Read the model definition and answer for the solid it produces. Units are mm, in the model's axes. Face numbers are marked on the shaded views. A direction names the side the tool comes from. Give positions to 0.01 mm unless a question says otherwise; leave off trailing zeros. Loops run counter-clockwise (first coordinate to the right, second up) from the corner with the lowest first, then second, coordinate; pieces in that order, holes last. Notation, with made-up numbers: (59.5, 16) -> (106.5, 16) arc R23 ccw to (106.5, 32) -> close; hole circle Ø9 at (-7.5, 67). An arc over 180 degrees is marked (long way). Write each question's results on one line, items separated by ' | '. Start each with the question number.
Item 1: Each of these flat-tipped pins is pushed along its axis until it touches: P1, Ø2, axis at x = 1.5, z = 2.5, coming from the +Y side; P2, Ø0.5, axis at y = 2.5, z = -3.5, coming from the -X side. Where does it stop, or does it pass through?
Item 2: Find the intervals of material crossed by line 1 (Z direction, x = 4, y = 1.85); line 2 (Z direction, x = -1, y = 2.45); line 3 (Y direction, x = 1.75, z = -2.5), in increasing order.
Item 3: Section A-A on z = -2 is taken. Write down the section's boundary in (x, y).
Item 4: Section B-B on y = 2.3 is taken. Write down the section's boundary in (x, z), and give its area (3 significant figures).
Item 5: Which of the six approach directions +Z, -Z, +X, -X, +Y, -Y give full straight-line access (tool end or side, diameter ignored) to the marked faces 1 and 2?
Item 6: Section C-C on x = 4 is taken. Write down the section's boundary in (y, z).
Item 7: Section D-D on z = 2.5 is taken. Write down the section's boundary in (x, y), and give its area (3 significant figures).
Item 8: Determine the mould class of the marked faces 3, 4 and 5 for opening direction Z: +Z half, -Z half, draft (parallel to the pull), parting line (faces both ways), or undercut.
Autodesk Inventor part; units mm, degrees
ref_plane "YZ Plane" through (0, 0, 0) normal (1, 0, 0) x (0, 1, 0)
ref_plane "XZ Plane" through (0, 0, 0) normal (0, 1, 0) x (-1, 0, 0)
ref_plane "XY Plane" through (0, 0, 0) normal (0, 0, 1) x (1, 0, 0)
sketch "草圖1" plane through (0, 0, 0) normal (0, 1, 0) x (-1, 0, 0)
  line L0 (2.7779, 3.5245) -> (-4.7221, 3.5245)
  line L1 (-4.7221, 3.5245) -> (-4.7221, -6.4755)
  line L2 (-4.7221, -6.4755) -> (2.7779, -6.4755)
  line L3 (2.7779, -6.4755) -> (2.7779, 3.5245)
  line L4 (1.1026, 3.5245) -> (1.1026, -6.4755)
  line L5 (1.1026, 0.7245) -> (-4.7221, 0.7245)
  line L6 (1.1026, -0.0755) -> (-4.7221, -0.0755)
  line L7 (1.1026, -2.8755) -> (-4.7221, -2.8755)
  line L8 (1.1026, -3.6755) -> (-4.7221, -3.6755)
  line L9 (1.1026, -1.4755) -> (-4.7221, -1.4755)
  line L10 (0.6975, -1.6358) -> (-3.8571, -1.6358)
  line L11 (-3.8571, -1.6358) -> (-3.8571, -2.7441)
  line L12 (-3.8571, -2.7441) -> (0.6975, -2.7441)
  line L13 (0.6975, -2.7441) -> (0.6975, -1.6358)
  line L14 (0.6975, -1.3152) -> (-3.8571, -1.3152)
  line L15 (-3.8571, -1.3152) -> (-3.8571, -0.207)
  line L16 (-3.8571, -0.207) -> (0.6975, -0.207)
  line L17 (0.6975, -0.207) -> (0.6975, -1.3152)
  line L18 (1.4446, 3.5245) -> (1.4446, -6.4755)
  line L19 (1.2626, 3.5245) -> (1.2626, -6.4755)
  line L20 (1.6046, 3.5245) -> (1.6046, -6.4755)
  line L21 (1.9385, 3.5245) -> (1.9385, -6.4755)
  line L22 (1.7785, 3.5245) -> (1.7785, -6.4755)
  line L23 (2.106, 3.5245) -> (2.106, -6.4755)
  line L24 (2.266, 3.5245) -> (2.266, -6.4755)
  line L25 (2.6263, 3.5245) -> (2.6263, -6.4755)
  line L26 (2.4663, 3.5245) -> (2.4663, -6.4755)
  line L27 (-3.8571, -0.207) -> (-3.8571, -1.3152)
  line L28 (-3.8571, -1.3152) -> (-4.7221, -1.3152)
  line L29 (-4.7221, -1.3152) -> (-4.7221, -0.207)
  line L30 (-4.7221, -0.207) -> (-3.8571, -0.207)
  line L31 (-3.8571, -1.6358) -> (-3.8571, -2.7441)
  line L32 (-3.8571, -2.7441) -> (-4.7221, -2.7441)
  line L33 (-4.7221, -2.7441) -> (-4.7221, -1.6358)
  line L34 (-4.7221, -1.6358) -> (-3.8571, -1.6358)
  line L35 (-3.8571, -0.207) -> (-3.8571, -1.3152)
  line L36 (-3.8571, -1.3152) -> (-4.7221, -1.3152)
  line L37 (-4.7221, -1.3152) -> (-4.7221, -0.207)
  line L38 (-4.7221, -0.207) -> (-3.8571, -0.207)
  line L39 (-3.8571, -1.6358) -> (-3.8571, -2.7441)
  line L40 (-3.8571, -2.7441) -> (-4.7221, -2.7441)
  line L41 (-4.7221, -2.7441) -> (-4.7221, -1.6358)
  line L42 (-4.7221, -1.6358) -> (-3.8571, -1.6358)
  point P0 (0, 0)
  dimension "d0" = 7.5
  dimension "d1" = 10
  dimension "d2" = 0.8
  dimension "d3" = 0.8
  dimension "d4" = 2.8
  dimension "d5" = 2.8
  dimension "d14" = 0.16
  dimension "d15" = 1.6753
  dimension "d16" = 0.16
  dimension "d17" = 0.16
  dimension "d18" = 0.16
  dimension "d19" = 0.16
extrude "擠出1" add sketch "草圖1" along normal blind 2 contours L3 L2 L25 L0 | L26 L2 L24 L0 | L23 L2 L21 L0 | L22 L2 L20 L0 | L18 L2 L19 L0 | L4 L5 L1 L0 | L2 L1 L8 L4
extrude "擠出2" add sketch "草圖1" along normal blind 2.5 contours L4 L6 L1 L5 | L8 L1 L7 L4
extrude "擠出3" add sketch "草圖1" along normal blind 2 contours L4 L9 L1 L28 L14 L17 L16 L30 L6 | L4 L7 L1 L32 L12 L13 L10 L34 L9
extrude "擠出4" add sketch "草圖1" along normal blind 1.8 contours L30 L15 L28 L1 | L16 L17 L14 L15 | L34 L11 L32 L1 | L10 L13 L12 L11
extrude "擠出5" add sketch "草圖1" along normal blind 2.05 contours L25 L2 L26 L0 | L24 L2 L23 L0 | L21 L2 L22 L0 | L20 L2 L18 L0 | L19 L2 L4 L0
properties part number "門"
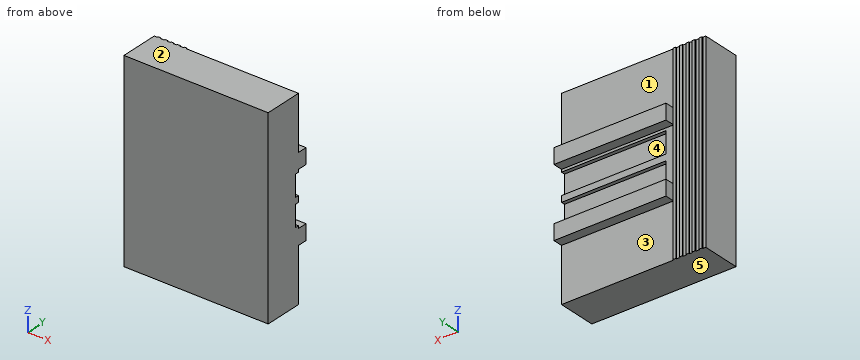
Findings:
1) P1: y = 2 | P2: x = -1.1
2) line 1: -6.48 to -2.74, -1.64 to -1.32, -0.21 to 3.52 | line 2: -3.68 to -2.88, -0.08 to 0.72 | line 3: 0 to 1.8
3) outline: (-2.78, 0) -> (4.72, 0) -> (4.72, 1.8) -> (-0.7, 1.8) -> (-0.7, 2) -> (-1.1, 2) -> (-1.1, 2.05) -> (-1.26, 2.05) -> (-1.26, 2) -> (-1.44, 2) -> (-1.44, 2.05) -> (-1.6, 2.05) -> (-1.6, 2) -> (-1.78, 2) -> (-1.78, 2.05) -> (-1.94, 2.05) -> (-1.94, 2) -> (-2.11, 2) -> (-2.11, 2.05) -> (-2.27, 2.05) -> (-2.27, 2) -> (-2.47, 2) -> (-2.47, 2.05) -> (-2.63, 2.05) -> (-2.63, 2) -> (-2.78, 2) -> close
4) outline: (-1.1, -3.68) -> (4.72, -3.68) -> (4.72, -2.88) -> (-1.1, -2.88) -> close; (-1.1, -0.08) -> (4.72, -0.08) -> (4.72, 0.72) -> (-1.1, 0.72) -> close | area: 9.32 mm2
5) face 1: +Z, +X, +Y | face 2: +Z, +X, -X, +Y, -Y
6) outline: (0, -6.48) -> (2, -6.48) -> (2, -3.68) -> (2.5, -3.68) -> (2.5, -2.88) -> (2, -2.88) -> (2, -2.74) -> (1.8, -2.74) -> (1.8, -1.64) -> (2, -1.64) -> (2, -1.32) -> (1.8, -1.32) -> (1.8, -0.21) -> (2, -0.21) -> (2, -0.08) -> (2.5, -0.08) -> (2.5, 0.72) -> (2, 0.72) -> (2, 3.52) -> (0, 3.52) -> close
7) outline: (-2.78, 0) -> (4.72, 0) -> (4.72, 2) -> (-1.1, 2) -> (-1.1, 2.05) -> (-1.26, 2.05) -> (-1.26, 2) -> (-1.44, 2) -> (-1.44, 2.05) -> (-1.6, 2.05) -> (-1.6, 2) -> (-1.78, 2) -> (-1.78, 2.05) -> (-1.94, 2.05) -> (-1.94, 2) -> (-2.11, 2) -> (-2.11, 2.05) -> (-2.27, 2.05) -> (-2.27, 2) -> (-2.47, 2) -> (-2.47, 2.05) -> (-2.63, 2.05) -> (-2.63, 2) -> (-2.78, 2) -> close | area: 15.0 mm2
8) face 3: draft | face 4: undercut | face 5: -Z half
